Read the model definition and answer for the solid it produces. Units are mm, in the model's axes. Face numbers are marked on the shaded views. A direction names the side the tool comes from. Give positions to 0.01 mm unless a question says otherwise; leave off trailing zeros. Loops run counter-clockwise (first coordinate to the right, second up) from the corner with the lowest first, then second, coordinate; pieces in that order, holes last. Notation, with made-up numbers: (29, 85.25) - (61, 85.25) arc R25 ccw to (61, 123.25) - close; hole circle Ø2 at (-16.5, 55.25). An arc over 180 degrees is marked (long way). Write each question's results on one line, items separated by ' | '. Start each with the question number.
Q1. Determine the mould class of the marked faces 1, 2, 3 and 4 for opening direction Y: +Y half, -Y half, draft (parallel to the pull), parting line (faces both ways), or undercut.
Q2. The part is cut by section C-C, the plane z = -14. Write down the section's boundary in (x, y).
Q3. For the marked faces 5, 6 and 7, determine the directions among +Z, -Z, +X, -X, +Y, -Y from which every point of the face is accessible in a straight line to the end or side of a thin tool.
Q4. The part is cut by section A-A, the plane y = 0. Write down the section's boundary in (x, z), plus the area to 3 significant figures.
Q5. Find the intervals of material crossed by line 1 (Y direction, x = -5, z = 0); line 2 (X direction, y = -2.25, z = 0); line 3 (Z direction, x = -6, y = -7), in increasing order. Write a range as from..to.
Q6. The part is cut by section D-D, the plane x = -2. Write down the section's boundary in (y, z), plus the area to 3 significant figures.
Q7. The part is cut by section B-B, the plane z = 0. State how many separate pieces and enclosed holes the cut face has, plus the area to 4 significant figures.
Q8. Given pin 1 (4 mm diameter, centred on x = 8, z = -3.5, fed in from -Y); pin 2 (8 mm diameter, centred on x = 41, y = 0.5, fed in from -Z); pin 3 (10 mm diameter, centred on y = 0.5, z = -12, fed in from +X), each flat-ended and moving along its own axis, determine where each tip first touches the part or whether it passes through.
```python
from build123d import *

# Parameters (mm, degrees)
BOSS_EXTRUDE3_DEPTH      = 60
BOSS_EXTRUDE3_DEPTH_BACK = 40
SKETCH1_R                = 25
SKETCH2_OUTSIDE_W        = 76.494
SKETCH2_OUTSIDE_H        = 76.494
SKETCH2_OUTSIDE_R        = 7.5
CUT_EXTRUDE3_DEPTH       = 60
SKETCH4_OUTSIDE_W        = 76.494
SKETCH4_OUTSIDE_H        = 76.494
SKETCH4_OUTSIDE_R        = 7.5
CUT_EXTRUDE4_DEPTH       = 30
SKETCH5_OUTSIDE_W        = 76.494
SKETCH5_OUTSIDE_H        = 76.494
SKETCH5_OUTSIDE_R        = 5
CUT_EXTRUDE5_DEPTH       = 35
CUT_EXTRUDE6_DEPTH       = 20
SKETCH7_R                = 2.5
CUT_EXTRUDE7_DEPTH       = 71.384657419
SKETCH8_R                = 4
CUT_EXTRUDE8_DEPTH       = 20
CUT_EXTRUDE10_DEPTH      = 5


with BuildPart() as part:
    # Sketch1 → Boss-Extrude3 (new, two sides: drawn at the far end of the back side and taken through both)
    with BuildSketch(Plane(origin=(0, 0, 0), x_dir=(0, 0, -1), z_dir=(1, 0, 0)).offset(-BOSS_EXTRUDE3_DEPTH_BACK)):
        Circle(SKETCH1_R)
    extrude(amount=BOSS_EXTRUDE3_DEPTH + BOSS_EXTRUDE3_DEPTH_BACK)

    # Sketch2 outside → Cut-Extrude3 (cut)
    with BuildSketch(Plane(origin=(60, 0, 0), x_dir=(0, 0, -1), z_dir=(1, 0, 0))):
        Rectangle(SKETCH2_OUTSIDE_W, SKETCH2_OUTSIDE_H)
        Circle(SKETCH2_OUTSIDE_R, mode=Mode.SUBTRACT)
    extrude(amount=-CUT_EXTRUDE3_DEPTH, mode=Mode.SUBTRACT)

    # Sketch4 outside → Cut-Extrude4 (cut)
    with BuildSketch(Plane.ZY.offset(40)):
        Rectangle(SKETCH4_OUTSIDE_W, SKETCH4_OUTSIDE_H)
        with Locations(Location((0, 0, 0), (0, 0, 180))):
            Circle(SKETCH4_OUTSIDE_R, mode=Mode.SUBTRACT)
    extrude(amount=-CUT_EXTRUDE4_DEPTH, mode=Mode.SUBTRACT)

    # Sketch5 outside → Cut-Extrude5 (cut)
    with BuildSketch(Plane(origin=(60, 0, 0), x_dir=(0, 0, -1), z_dir=(1, 0, 0))):
        Rectangle(SKETCH5_OUTSIDE_W, SKETCH5_OUTSIDE_H)
        Circle(SKETCH5_OUTSIDE_R, mode=Mode.SUBTRACT)
    extrude(amount=-CUT_EXTRUDE5_DEPTH, mode=Mode.SUBTRACT)

    # Sketch6 → Cut-Extrude6 (cut)
    with BuildSketch(Plane(origin=(60, 0, 0), x_dir=(0, 0, -1), z_dir=(1, 0, 0))):
        with BuildLine():
            Line((-4.582575695, 2), (4.582575695, 2))
            ThreePointArc((4.582575695, 2), (0, 5), (-4.582575695, 2))
        make_face()
    extrude(amount=-CUT_EXTRUDE6_DEPTH, mode=Mode.SUBTRACT)

    # Sketch7 → Cut-Extrude7 (cut, through all)
    with BuildSketch(Plane(origin=(0, 2, 0), x_dir=(1, 0, 0), z_dir=(0, 1, 0))):
        with Locations(Location((50, 0, 0), (0, 0, 270))):
            Circle(SKETCH7_R)
    extrude(amount=-CUT_EXTRUDE7_DEPTH, mode=Mode.SUBTRACT)

    # Sketch8 → Cut-Extrude8 (cut)
    with BuildSketch(Plane(origin=(0, 0, 0), x_dir=(0, 0, -1), z_dir=(1, 0, 0))):
        with Locations((0, 15)):
            Circle(SKETCH8_R)
        with Locations((12.990381057, -7.5)):
            Circle(SKETCH8_R)
        with Locations((-12.990381057, -7.5)):
            Circle(SKETCH8_R)
    extrude(amount=-CUT_EXTRUDE8_DEPTH, mode=Mode.SUBTRACT)

    # Sketch11 → Cut-Extrude10 (cut)
    with BuildSketch(Plane.ZY.offset(40)):
        with BuildLine():
            Line((7.071067812, 2.5), (-7.071067812, 2.5))
            ThreePointArc((-7.071067812, 2.5), (-7.5, 0), (-7.071067812, -2.5))
            Line((-7.071067812, -2.5), (7.071067812, -2.5))
            ThreePointArc((7.071067812, -2.5), (7.391989197, -1.26826484), (7.5, 0))
            ThreePointArc((7.5, 0), (7.391989197, 1.26826484), (7.071067812, 2.5))
        make_face()
    extrude(amount=-CUT_EXTRUDE10_DEPTH, mode=Mode.SUBTRACT)


solid = part.part
```
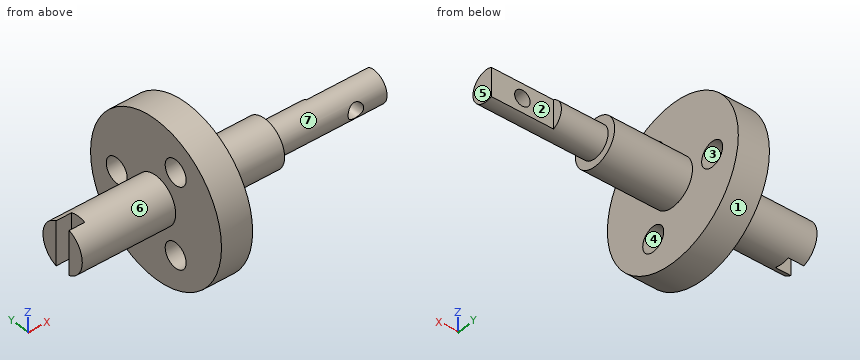
Check sheet entries:
1) face 1: parting line | face 2: +Y half | face 3: undercut | face 4: undercut
2) outline: (-10, -20.71) - (0, -20.71) - (0, -11.37) - (-10, -11.37) - close; (-10, -3.63) - (0, -3.63) - (0, 20.71) - (-10, 20.71) - close
3) face 5: +Z, -Z, +X, +Y, -Y | face 6: -X | face 7: +X
4) outline: (-35, -7.5) - (-10, -7.5) - (-10, -25) - (0, -25) - (0, -7.5) - (25, -7.5) - (25, -5) - (60, -5) - (60, 5) - (25, 5) - (25, 7.5) - (0, 7.5) - (0, 25) - (-10, 25) - (-10, 7.5) - (-35, 7.5) - close; hole circle Ø5 at (50, 0) | area: 1,580 mm^2
5) line 1: y = -25..11, 19..25 | line 2: x = -35..47.5, 52.5..60 | line 3: z = -24..-16.96, -9.02..9.02, 16.96..24
6) outline: circle Ø50 at (0, 0); hole circle Ø8 at (-7.5, -12.99); hole circle Ø8 at (-7.5, 12.99); hole circle Ø8 at (15, 0) | area: 1,810 mm^2
7) separate pieces: 3 | enclosed holes: 0 | area: 1,475 mm^2
8) pin 1: stops at y = -7.35 | pin 2: stops at z = -5 | pin 3: stops at x = 25
